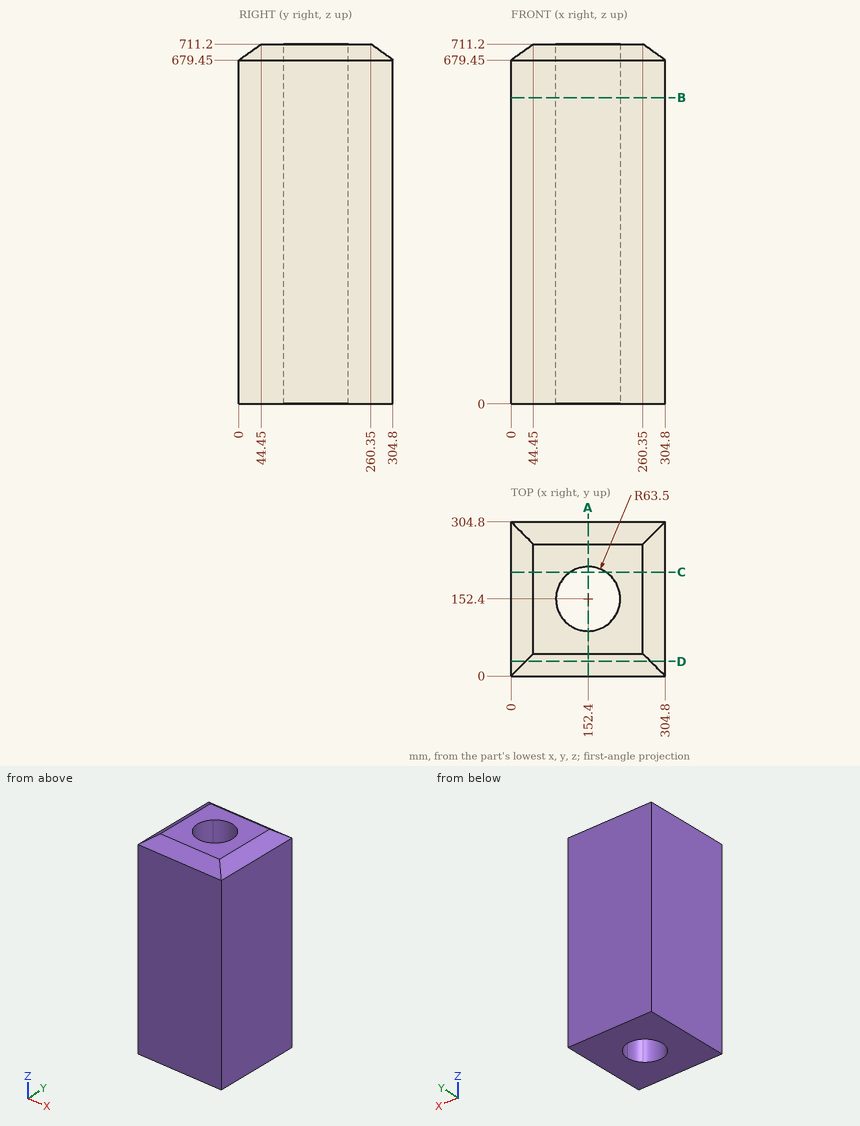
Here's the drawing with two shaded views (mm, measured from the low corner). I have some questions. Coordinates: 2 decimals unless noted, no trailing zeros. Order: outer loops, then holes, each group sorted by start corner. A loop starts at its lowest first (then second) coordinate and runs counter-clockwise, first axis right, second up.
Item 1: If we section it at B-B, the plane z = 605: List the corners of the cut face in (x, y) for me, then the cut area to 3 significant figures.
Response values:
outline: (0, 0) - (304.8, 0) - (304.8, 304.8) - (0, 304.8) - close; hole (197.3, 107.5) arc R63.5 ccw to (215.9, 152.4) arc R63.5 ccw (long way) to start
area: 80,200 mm2
Item 2: If we section it at A-A, the plane x = 152.4: List the corners of the cut face in (y, z) for me.
Response values:
outline: (0, 0) - (88.9, 0) - (88.9, 711.2) - (44.45, 711.2) - (0, 679.45) - close; (215.9, 0) - (304.8, 0) - (304.8, 679.45) - (260.35, 711.2) - (215.9, 711.2) - close
Item 3: If we section it at C-C, the plane y = 205.5: List the corners of the cut face in (x, z) for me.
Response values:
outline: (0, 0) - (117.58, 0) - (117.58, 711.2) - (44.45, 711.2) - (0, 679.45) - close; (187.22, 0) - (304.8, 0) - (304.8, 679.45) - (260.35, 711.2) - (187.22, 711.2) - close
Item 4: I'm going to push a flat-ended pin straight in: pin 1 Ø6 at (x, y) = (37.5, 208) entering from +Z. Where does the tip first touch, or does it pass through?
Response values:
pin 1: stops at z = 708.38
Item 5: If we section it at D-D, the plane y = 29: List the corners of the cut face in (x, z) for me, then the cut area to 3 significant figures.
Response values:
outline: (0, 0) - (304.8, 0) - (304.8, 679.45) - (275.8, 700.16) - (29, 700.16) - (0, 679.45) - close
area: 213,000 mm2
Item 6: I need wall thicknesses on probe 1 along X at (y, z) = (176.5, 203); probe 2 along X at (y, z) = (110, 485); probe 3 along Y at (x, z) = (103, 231.5). Which ranges of each line are inside material? Lowest first, please.
Response values:
probe 1: x = 0 to 93.65, 211.15 to 304.8
probe 2: x = 0 to 105.13, 199.67 to 304.8
probe 3: y = 0 to 112.5, 192.3 to 304.8
